```python
from build123d import *

# Parameters (mm, degrees)
F0_W     = 36.068
F0_H     = 4.0005
F1_DEPTH = 120.65
F4_D     = 6.7564


with BuildPart() as f1:
    # F0 (on Right) → F1 (new body)
    with BuildSketch(Plane.YZ):
        with Locations((18.034, 2.00025)):
            Rectangle(F0_W, F0_H)
    extrude(amount=-F1_DEPTH)

    # F4 (through all)
    with Locations(Plane.XY.offset(4.0005)):
        with Locations((-114.3, 26.543), (-114.3, 9.525)):
            Hole(F4_D / 2)


solid = f1.part
```
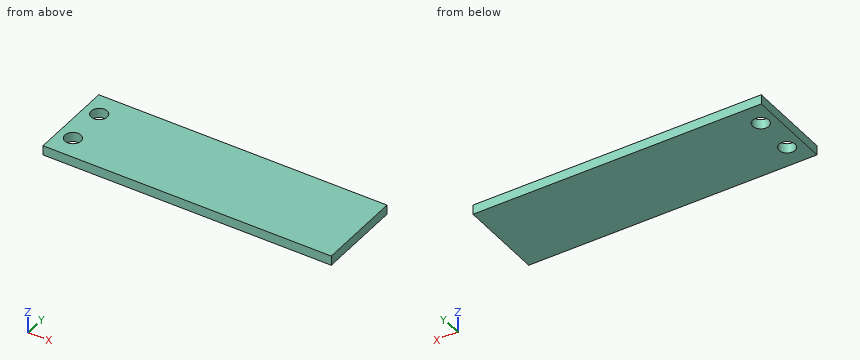
Could you check a few things on this model? Use its own coordinates, in mm. Coordinates: 2 decimals unless noted, no trailing zeros. Write each loop counter-clockwise with the first axis right and the second up, starting at its lowest first coordinate (ties: lowest second). Pieces come first, ordered by that corner, then holes. Notation, with made-up numbers: (21.25, 43) - (70.25, 43) arc R21 cw to (70.25, 59) - close; hole circle Ø6 at (70, 17). An arc over 180 degrees is marked (long way). Use a Markdown table: item, result.
Q1. Imagine slicing it at B-B (y = 28). List the corners of the cut face in (x, z) for me.
Geometry check:
| item | result |
|---|---|
| outline | (-120.65, 0) - (-117.35, 0) - (-117.35, 4) - (-120.65, 4) - close; (-111.25, 0) - (0, 0) - (0, 4) - (-111.25, 4) - close |
Q2. Imagine slicing it at A-A (x = -114.3). List the corners of the cut face in (y, z) for me.
Geometry check:
| item | result |
|---|---|
| outline | (0, 0) - (6.15, 0) - (6.15, 4) - (0, 4) - close; (12.9, 0) - (23.16, 0) - (23.16, 4) - (12.9, 4) - close; (29.92, 0) - (36.07, 0) - (36.07, 4) - (29.92, 4) - close |
Q3. Please list where these lines run through material, in increasing order: L1, parallel to Y at x = -114.3, z = 1.95; L2, parallel to X at y = 26.5, z = 3.8; L3, parallel to X at y = 10, z = 3.45.
Geometry check:
| item | result |
|---|---|
| L1 | y = 0 to 6.15, 12.9 to 23.16, 29.92 to 36.07 |
| L2 | x = -120.65 to -117.68, -110.92 to 0 |
| L3 | x = -120.65 to -117.64, -110.96 to 0 |
Q4. Imagine slicing it at C-C (z = 1.8). List the corners of the cut face in (x, y) for me (3 decimals), and give its area (3 significant figures).
Geometry check:
| item | result |
|---|---|
| outline | (-120.65, 0) - (0, 0) - (0, 36.068) - (-120.65, 36.068) - close; hole circle Ø6.756 at (-114.3, 9.525); hole circle Ø6.756 at (-114.3, 26.543) |
| area | 4,280 mm2 |
